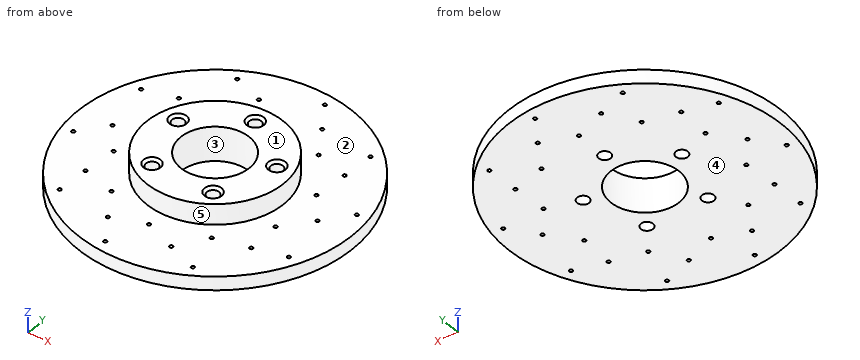
from build123d import *

# Parameters (mm, degrees)
F0_R           = 101.673036
F1_DEPTH       = 10.16
F2_R           = 50.825474
F3_DEPTH       = 15.24
F5_D           = 50.8
F7_D           = 8.89
F7_CSINK_D     = 12.7
F7_CSINK_ANGLE = 90
F9_D           = 2.54


with BuildPart() as f1:
    # F0 (on Top) → F1 (new body)
    with BuildSketch(Plane.XY):
        Circle(F0_R)
    extrude(amount=F1_DEPTH)

    # F2 (on face) → F3 (join)
    with BuildSketch(Plane.XY.offset(10.16)):
        Circle(F2_R)
    extrude(amount=F3_DEPTH)

    # F5 (through all)
    with Locations(Plane.XY.offset(25.4)):
        with Locations((0, 0)):
            Hole(F5_D / 2)

    # F7 (through all)
    with Locations(Plane.XY.offset(25.4)):
        with Locations((0, 38.806446), (-36.907123, 11.991851), (-22.809857, -31.395074), (22.809857, -31.395074), (36.907123, 11.991851)):
            CounterSinkHole(F7_D / 2, F7_CSINK_D / 2, counter_sink_angle=F7_CSINK_ANGLE)

    # F9 (through all)
    with Locations(Plane.XY.offset(10.16)):
        with Locations((10.266128, 92.69405), (-46.178724, 81.025341), (-23.668928, 72.845469), (0.032693, 63.665586), (23.668928, 72.845469), (37.448142, 51.487324), (62.789668, 68.956783), (61.966057, 45.020975), (60.559673, 19.642655), (91.329689, 18.880369), (76.594258, 0), (60.539468, -19.704841), (84.984873, -38.407705), (61.966057, -45.020975), (37.395243, -51.525757), (46.178724, -81.025341), (23.668928, -72.845469), (-0.032693, -63.665586), (-10.266128, -92.69405), (-23.668928, -72.845469), (-37.448142, -51.487324), (-62.789668, -68.956783), (-61.966057, -45.020975), (-60.559673, -19.642655), (-91.329689, -18.880369), (-76.594258, 0), (-60.539468, 19.704841), (-84.984873, 38.407705), (-61.966057, 45.020975), (-37.395243, 51.525757)):
            Hole(F9_D / 2)


solid = f1.part
Geometry: final body of the model. Coordinates: model frame, mm. Face numbers are marked on the shaded views. A direction names the side the tool comes from. Round coordinates to 2 decimals unless told otherwise and drop trailing zeros. Loops run counter-clockwise (first coordinate to the right, second up) from the corner with the lowest first, then second, coordinate; pieces in that order, holes last. Notation, with made-up numbers: M 29,-8 L 65,-8 A24 cw 65,13 Z; hole C 18.5,-16.5 d6. An arc over 180 degrees is marked long. One line per question, with ' | ' between items.
(1) Pull-direction query (Y, two-part tool) for the marked faces 3, 4 and 5; classes: +Y half, -Y half, draft (parallel to the pull), parting line (faces both ways), or undercut.
Check result:
face 3: undercut | face 4: draft | face 5: parting line
(2) Cut plane A-A on z = 15.25. Return the cut outline in (x, y) (3 decimals).
Check result:
outline: C 0,0 d101.651; hole C -36.907,11.992 d8.89; hole C -22.81,-31.395 d8.89; hole C 0,0 d50.8; hole C 0,38.806 d8.89; hole C 22.81,-31.395 d8.89; hole C 36.907,11.992 d8.89
(3) Material intervals for line 1 along Y through (x, z) = (0, 17.5); line 2 along Y through (x, z) = (21, 18); line 3 along Z through (x, y) = (-41.5, -36), sorted ascending. Write a range as from..to.
Check result:
line 1: y = -50.83..-25.4, 25.4..34.36, 43.25..50.83 | line 2: y = -46.28..-35.45, -27.34..-14.29, 14.29..46.28 | line 3: z = 0..10.16
(4) Access query for the marked faces 1 and 2. Directions: +Z, -Z, +X, -X, +Y, -Y. A direction counts if a zero-diameter tool reaches every point of the face in a straight line with its end or side. Return the directions, or none.
Check result:
face 1: +Z, +X, -X, +Y, -Y | face 2: +Z
(5) Cut plane B-B on y = -60. Return the cut outline in (x, z), plus the area to 3 significant figures.
Check result:
outline: M -82.08,0 L 82.08,0 L 82.08,10.16 L -82.08,10.16 Z | area: 1,670 mm2
(6) Contact query for flat-ended pins moving along their axis: P1, Ø10, axis at x = -22.81, y = -31.4, coming from the +Z side; P2, Ø1, axis at y = 44, z = 13, coming from the -X side; P3, Ø4, axis at x = -10.27, y = -92.69, coming from the +Z side. Output: stop coordinate, or through.
Check result:
P1: stops at z = 24.05 | P2: stops at x = -26.29 | P3: stops at z = 10.16
